The model under review builds one solid part; all positions refer to its coordinate system, in mm. A direction names the side the tool comes from. Round coordinates to 2 decimals unless told otherwise and drop trailing zeros. Use a Markdown table: item, result. Add a question column.
1. The part is to be moulded in two halves that separate along Y. For faces 1 (the flat face through (-8.6, 7.1, 172.6)), 2 (the flat face through (-11, 20, 173)), 3 (the flat face through (3, -2, 350)), say which applies: +Y half, -Y half, draft (parallel to the pull), parting line (faces both ways), or undercut.
2. To check wall thickness, follow probe 1 along Y at (x, z) = (-14, 71); probe 2 along X at (y, z) = (4, 256). State the ranges of each line that lie inside material, in increasing order.
3. Consider section A-A on z = 272. Count the separate pieces of the cut face and the enclosed holes in it, then the cut area to 3 significant figures.
4. Insertion check: P1, Ø5.5, axis at x = -16, z = 242, coming from the -Y side; P2, Ø9, axis at x = -1.5, z = 164.5, coming from the -Y side; P3, Ø1.1, axis at y = 19.5, z = 143, coming from the +X side; P4, Ø0.8, axis at y = -3.5, z = 202.5, coming from the -X side. Each pin has a flat end and moves straight along its axis. Give the tip position at first contact, or say it passes through.
5. For faces 4 (the flat face through (-11.69, 15, 173)), 5 (the flat face through (3, -2, 0)), 6 (the flat face through (0, 5.5, 173)), list the 3-axis set-ups (+Z, -Z, +X, -X, +Y, -Y) from which the entire face can be reached by the end or side of a thin tool; tool diameter is ignored.
from build123d import *
from build123d.topology import SkipClean

# Parameters (mm, degrees)
BOSS_EXTRUDE1_DEPTH  = 350
MIRROR3_COPY_1_DEPTH = 350
MIRROR3_COPY_2_DEPTH = 350


with BuildPart() as part:
    # Sketch1 → Boss-Extrude1 (new body)
    with BuildSketch(Plane.XY):
        with BuildLine():
            Line((3.4, 0), (5.5, 0))
            Line((5.5, 0), (5.5, 4))
            Line((5.5, 4), (11.69, 10.19))
            Line((11.69, 10.19), (18.2, 10.19))
            Line((18.2, 10.19), (18.2, 5.265595036))
            Line((18.2, 5.265595036), (15.5, 5.265595036))
            Line((15.5, 5.265595036), (15.5, 2.965595036))
            Line((15.5, 2.965595036), (19, 2.965595036))
            Line((19, 2.965595036), (19, 3.965595036))
            Line((19, 3.965595036), (20, 3.965595036))
            Line((20, 3.965595036), (20, 15.5))
            ThreePointArc((20, 15.5), (18.681980515, 18.681980515), (15.5, 20))
            Line((15.5, 20), (6.385304712, 20))
            Line((6.385304712, 20), (6.385304712, 19))
            Line((6.385304712, 19), (5.385304712, 19))
            Line((5.385304712, 19), (5.385304712, 15.5))
            Line((5.385304712, 15.5), (7.685304712, 15.5))
            Line((7.685304712, 15.5), (7.685304712, 18.2))
            Line((7.685304712, 18.2), (10.19, 18.2))
            Line((10.19, 18.2), (10.19, 11.69))
            Line((10.19, 11.69), (4, 5.5))
            Line((4, 5.5), (0, 5.5))
            Line((0, 5.5), (0, 3.4))
            ThreePointArc((0, 3.4), (2.404163056, 2.404163056), (3.4, 0))
        make_face()
        with BuildLine():
            Line((18.5, 11.69), (18.5, 15.5))
            ThreePointArc((18.5, 15.5), (17.621320344, 17.621320344), (15.5, 18.5))
            Line((15.5, 18.5), (11.69, 18.5))
            Line((11.69, 18.5), (11.69, 11.69))
            Line((11.69, 11.69), (18.5, 11.69))
        make_face(mode=Mode.SUBTRACT)
    boss_extrude1 = extrude(amount=BOSS_EXTRUDE1_DEPTH)

    # Mirror1: Boss-Extrude1 across plane
    add(boss_extrude1.mirror(Plane.ZX))

    # Mirror2: Boss-Extrude1 across plane
    add(boss_extrude1.mirror(Plane(origin=(0, 0, 0), x_dir=(0, 0, 1), z_dir=(1, 0, 0))))

    # Mirror3 copy 1 sketch → Mirror3 copy 1 (add)
    with BuildSketch(Plane(origin=(0, 0, 0), x_dir=(-1, 0, 0), z_dir=(0, 0, 1))):
        with BuildLine():
            Line((3.4, 0), (5.5, 0))
            Line((5.5, 0), (5.5, 4))
            Line((5.5, 4), (11.69, 10.19))
            Line((11.69, 10.19), (18.2, 10.19))
            Line((18.2, 10.19), (18.2, 5.265595036))
            Line((18.2, 5.265595036), (15.5, 5.265595036))
            Line((15.5, 5.265595036), (15.5, 2.965595036))
            Line((15.5, 2.965595036), (19, 2.965595036))
            Line((19, 2.965595036), (19, 3.965595036))
            Line((19, 3.965595036), (20, 3.965595036))
            Line((20, 3.965595036), (20, 15.5))
            ThreePointArc((20, 15.5), (18.681980515, 18.681980515), (15.5, 20))
            Line((15.5, 20), (6.385304712, 20))
            Line((6.385304712, 20), (6.385304712, 19))
            Line((6.385304712, 19), (5.385304712, 19))
            Line((5.385304712, 19), (5.385304712, 15.5))
            Line((5.385304712, 15.5), (7.685304712, 15.5))
            Line((7.685304712, 15.5), (7.685304712, 18.2))
            Line((7.685304712, 18.2), (10.19, 18.2))
            Line((10.19, 18.2), (10.19, 11.69))
            Line((10.19, 11.69), (4, 5.5))
            Line((4, 5.5), (0, 5.5))
            Line((0, 5.5), (0, 3.4))
            ThreePointArc((0, 3.4), (2.404163056, 2.404163056), (3.4, 0))
        make_face()
        with BuildLine():
            Line((18.5, 11.69), (18.5, 15.5))
            ThreePointArc((18.5, 15.5), (17.621320344, 17.621320344), (15.5, 18.5))
            Line((15.5, 18.5), (11.69, 18.5))
            Line((11.69, 18.5), (11.69, 11.69))
            Line((11.69, 11.69), (18.5, 11.69))
        make_face(mode=Mode.SUBTRACT)
    extrude(amount=MIRROR3_COPY_1_DEPTH)

    # Mirror3 copy 2 sketch → Mirror3 copy 2 (add)
    with SkipClean():  # the faces are left unmerged after this step: merging them gives an invalid solid
        with BuildSketch(Plane.XY):
            with BuildLine():
                Line((3.4, 0), (5.5, 0))
                Line((5.5, 0), (5.5, -4))
                Line((5.5, -4), (11.69, -10.19))
                Line((11.69, -10.19), (18.2, -10.19))
                Line((18.2, -10.19), (18.2, -5.265595036))
                Line((18.2, -5.265595036), (15.5, -5.265595036))
                Line((15.5, -5.265595036), (15.5, -2.965595036))
                Line((15.5, -2.965595036), (19, -2.965595036))
                Line((19, -2.965595036), (19, -3.965595036))
                Line((19, -3.965595036), (20, -3.965595036))
                Line((20, -3.965595036), (20, -15.5))
                ThreePointArc((20, -15.5), (18.681980515, -18.681980515), (15.5, -20))
                Line((15.5, -20), (6.385304712, -20))
                Line((6.385304712, -20), (6.385304712, -19))
                Line((6.385304712, -19), (5.385304712, -19))
                Line((5.385304712, -19), (5.385304712, -15.5))
                Line((5.385304712, -15.5), (7.685304712, -15.5))
                Line((7.685304712, -15.5), (7.685304712, -18.2))
                Line((7.685304712, -18.2), (10.19, -18.2))
                Line((10.19, -18.2), (10.19, -11.69))
                Line((10.19, -11.69), (4, -5.5))
                Line((4, -5.5), (0, -5.5))
                Line((0, -5.5), (0, -3.4))
                ThreePointArc((0, -3.4), (2.404163056, -2.404163056), (3.4, 0))
            make_face()
            with BuildLine():
                Line((18.5, -11.69), (18.5, -15.5))
                ThreePointArc((18.5, -15.5), (17.621320344, -17.621320344), (15.5, -18.5))
                Line((15.5, -18.5), (11.69, -18.5))
                Line((11.69, -18.5), (11.69, -11.69))
                Line((11.69, -11.69), (18.5, -11.69))
            make_face(mode=Mode.SUBTRACT)
        extrude(amount=MIRROR3_COPY_2_DEPTH)


solid = part.part
Answer block:
| question | item | result |
|---|---|---|
| 1 | face 1 | undercut |
| 1 | face 2 | +Y half |
| 1 | face 3 | draft |
| 2 | probe 1 | -20 to -18.5, -11.69 to -10.19, 10.19 to 11.69, 18.5 to 20 |
| 2 | probe 2 | -20 to -15.5, -5.5 to 5.5, 15.5 to 20 |
| 3 | separate pieces | 1 |
| 3 | enclosed holes | 5 |
| 3 | area | 468 mm^2 |
| 4 | P1 | y = -20 |
| 4 | P2 | y = -19 |
| 4 | P3 | x = 18.39 |
| 4 | P4 | x = -19 |
| 5 | face 4 | +Z, -Z |
| 5 | face 5 | -Z, +X, -X, +Y, -Y |
| 5 | face 6 | +Z, -Z, +Y |
